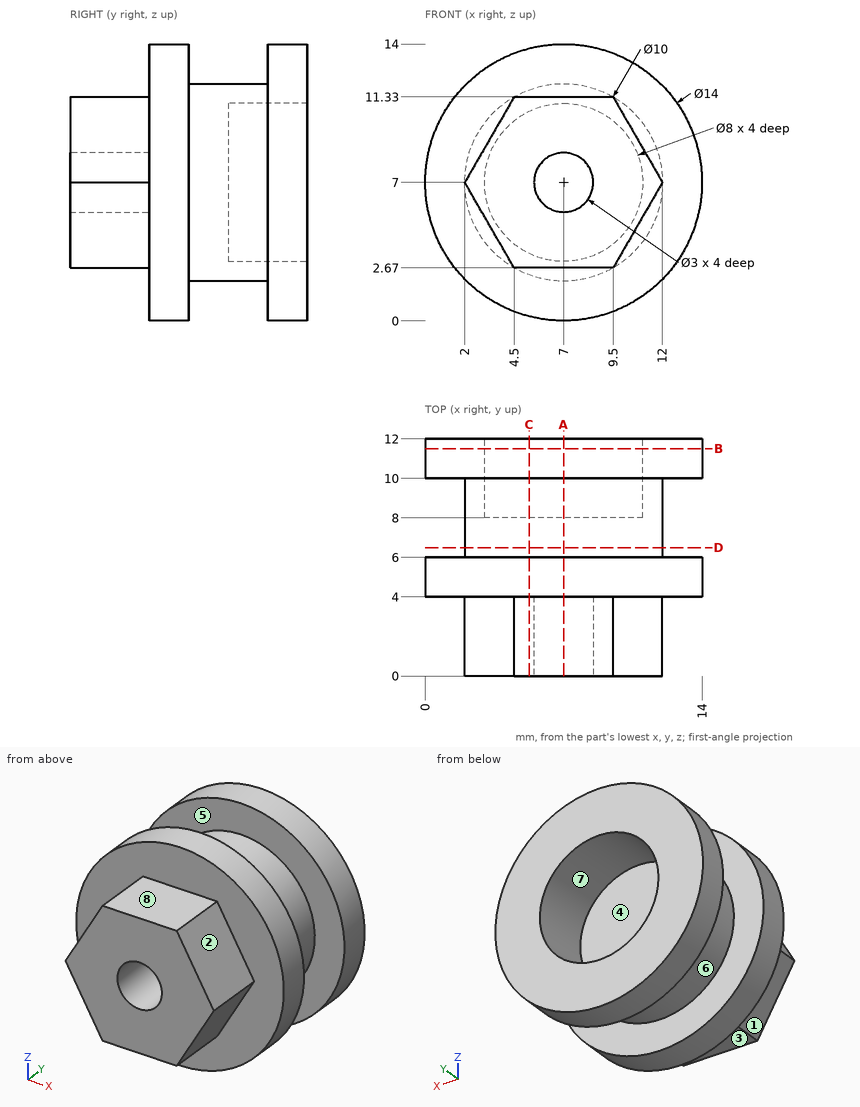
Print and shaded views of the part. All mm, measured from the part's lowest x, y and z. A direction names the side the tool comes from. Round coordinates to 2 decimals unless told otherwise and drop trailing zeros. Write each loop counter-clockwise with the first axis right and the second up, starting at its lowest first coordinate (ties: lowest second). Pieces come first, ordered by that corner, then holes.
(1) Probe line 1 along Y through (x, z) = (12.5, 8.75); line 2 along X through (y, z) = (10.8, 7); line 3 along Y through (x, z) = (4.5, 8.5). List the from-to ranges inside material, lowest first.
(2) Slice it at B-B, the plane y = 11.5. Write the cut outline in (x, z), and give its area (3 significant figures).
(3) 3-axis set-ups, long thin cutter, end or side, ignore diameter. For the marked faces 1, 2, 3, 4 and 5: which of +Z, -Z, +X, -X, +Y, -Y reach the whole face in a straight line?
(4) Mould opens along Z. For the marked faces 6, 7 and 8 say: pulls with the +Z half, pulls with the -Z half, needs draft (parallel to the pull), parting line crosses it, or undercut.
(5) Slice it at D-D, the plane y = 6.5. Write the cut outline in (x, z), and give its area (3 significant figures).
(6) Slice it at A-A, the plane x = 7. Write the cut outline in (y, z).
(7) Slice it at C-C, the plane x = 5.25. Write the cut outline in (y, z).
(8) Drop flat-ended pins along their axis: P1, Ø3, axis at y = 1, z = 10.5, coming from the -X side (1 decimal); P2, Ø1, axis at x = 4.5, y = 8.5, coming from the -Z side; P3, Ø2, axis at x = 6.5, z = 6.5, coming from the +Y side. Give the stop position or say it passes through.
From the geometry:
1. line 1: y = 4 to 6, 10 to 12
1. line 2: x = 0 to 3, 11 to 14
1. line 3: y = 0 to 8
2. outline: circle Ø14 at (7, 7); hole circle Ø8 at (7, 7)
2. area: 104 mm2
3. face 1: -Z, -X, -Y
3. face 2: +Z, +X, -Y
3. face 3: -Z, +X, -X, -Y
3. face 4: +Y
3. face 5: none
4. face 6: parting line crosses it
4. face 7: undercut
4. face 8: pulls with the +Z half
5. outline: circle Ø10 at (7, 7)
5. area: 78.5 mm2
6. outline: (0, 2.67) - (4, 2.67) - (4, 0) - (6, 0) - (6, 2) - (10, 2) - (10, 0) - (12, 0) - (12, 3) - (8, 3) - (8, 11) - (12, 11) - (12, 14) - (10, 14) - (10, 12) - (6, 12) - (6, 14) - (4, 14) - (4, 11.33) - (0, 11.33) - (0, 8.5) - (4, 8.5) - (4, 5.5) - (0, 5.5) - close
7. outline: (0, 2.67) - (4, 2.67) - (4, 0.22) - (6, 0.22) - (6, 2.32) - (10, 2.32) - (10, 0.22) - (12, 0.22) - (12, 3.4) - (8, 3.4) - (8, 10.6) - (12, 10.6) - (12, 13.78) - (10, 13.78) - (10, 11.68) - (6, 11.68) - (6, 13.78) - (4, 13.78) - (4, 11.33) - (0, 11.33) - close
8. P1: stops at x = 3.2
8. P2: stops at z = 2.42
8. P3: stops at y = 8
